```python
from build123d import *

# Parameters (mm, degrees)
F1_DEPTH = 16.256
F2_R     = 5.08
F3_W     = 14.0684605576
F3_H     = 6.096
F4_DEPTH = 10.668
F5_R     = 5.08
F6_R     = 4.8101644532
F7_DEPTH = 25.4


with BuildPart() as f1:
    # F0 (on Top) → F1 (new body)
    with BuildSketch(Plane.XY):
        Polygon((26.3900562345, 4.9985722308), (3.4010511667, 26.6430787142), (-24.288091016, 11.4677559795), (-18.4119169365, -19.5556157441), (12.9089005512, -23.5537911803), align=None)
    extrude(amount=F1_DEPTH)

    # F2
    f2_edges = [f1.edges().sort_by_distance(p)[0] for p in [
        (-18.411917, -19.555616, 8.128),
        (-2.751508, -21.554703, 0),
        (-2.751508, -21.554703, 16.256),
        (-21.350004, -4.04393, 0),
        (-10.44352, 19.055417, 0),
        (14.895554, 15.820825, 0),
        (19.649478, -9.277609, 0),
        (19.649478, -9.277609, 16.256),
        (14.895554, 15.820825, 16.256),
        (-10.44352, 19.055417, 16.256),
        (-21.350004, -4.04393, 16.256),
        (3.401051, 26.643079, 8.128),
        (-24.288091, 11.467756, 8.128),
        (12.908901, -23.553791, 8.128),
        (26.390056, 4.998572, 8.128),
    ]]
    fillet(f2_edges, radius=F2_R)

    # F3 (on face) → F4 (join)
    with BuildSketch(Plane(origin=(-21.3500039762, -4.0439298823, 0), x_dir=(0.1861022589, -0.9825303808, 0), z_dir=(-0.9825303808, -0.1861022589, 0))):
        with Locations((0.7629252505, 8.128)):
            Rectangle(F3_W, F3_H)
    extrude(amount=F4_DEPTH)

    # F5
    f5_edges = [f1.edges().sort_by_distance(p)[0] for p in [
        (-30.38057, -13.690211, 8.128),
        (-32.998742, 0.132479, 8.128),
    ]]
    fillet(f5_edges, radius=F5_R)

    # F6 (on face) → F7 (cut)
    with BuildSketch(Plane.XY.offset(11.176)):
        with Locations((-26.1089652777, -5.1103131846)):
            Circle(F6_R)
    extrude(amount=-F7_DEPTH, mode=Mode.SUBTRACT)


solid = f1.part
```
The model under review builds one solid part; all positions refer to its coordinate system, in mm. A direction names the side the tool comes from. Give positions to 0.01 mm unless a question says otherwise; leave off trailing zeros. Write each loop counter-clockwise with the first axis right and the second up, starting at its lowest first coordinate (ties: lowest second). Pieces come first, ordered by that corner, then holes. Notation, with made-up numbers: (63.5, 72.25) - (120.5, 72.25) arc R8 cw to (120.5, 80.25) - close; hole circle Ø1 at (21.25, -24.75). An arc over 180 degrees is marked (long way). Answer in a Markdown table with one row per item. Add a question column.
1. Draft analysis for pull direction Y (two halves, no side actions). For faces 1 (the cylindrical face through (13.779, 14.882, 1.528)), 2 (the flat face through (-23.067, 5.02, 8.085)), 3 (the cylindrical face through (-19.9, -3.94, 1.53)), state which applies: +Y half, -Y half, draft (parallel to the pull), parting line (faces both ways), or undercut.
2. We need section A-A on z = 9.75. Write out the cut boundary in (x, y).
3. Tool access review of faces 4 (the flat face through (-22, -8, 5.08)), 5 (the flat face through (-22, -8, 11.176)), 6 (the flat face through (-22.61, -12.22, 8.09)), 7 (the flat face through (-25.224, 1.605, 8.085)): name each direction out of +Z, -Z, +X, -X, +Y, -Y from which nothing blocks a thin tool from reaching the whole face with its end or side.
4. Insertion check: P1, Ø4, axis at y = -9.5, z = 12.5, coming from the +X side; P2, Ø1, axis at y = -9.5, z = 2, coming from the +X side; P3, Ø3.5, axis at x = -25, y = -8.5, coming from the +Z side. Each pin has a flat end and moves straight along its axis. Give the tip position at first contact, or say it passes through.
5. Wall thickness on line 1 along Y through (x, z) = (-25.5, 7.25); line 2 along Y through (x, z) = (-4.5, 2.5); line 3 along Y through (x, z) = (-6, 1.25): over which ranges is each line inside the solid? List them lowest first. Write a range as [from, to].
6. We need section B-B on z = 13.25. Write out the cut boundary in (x, y).
Ans:
| question | item | result |
|---|---|---|
| 1 | face 1 | +Y half |
| 1 | face 2 | undercut |
| 1 | face 3 | -Y half |
| 2 | outline | (-32.05, -4.86) - (-31.33, -8.7) arc R5.08 ccw to (-25.39, -12.74) - (-19.9, -11.7) - (-19.1, -15.93) arc R5.08 ccw to (-14.75, -20.02) - (9.25, -23.09) arc R5.08 ccw to (14.48, -20.22) - (24.81, 1.66) arc R5.08 ccw to (23.7, 7.53) - (6.09, 24.11) arc R5.08 ccw to (0.16, 24.87) - (-21.05, 13.24) arc R5.08 ccw to (-23.6, 7.84) - (-22.52, 2.12) - (-28.01, 1.08) arc R5.08 ccw to start; hole circle Ø9.62 at (-26.11, -5.11) |
| 3 | face 4 | -Z, -X, -Y |
| 3 | face 5 | +Z, -X, -Y |
| 3 | face 6 | +Z, -Z, -Y |
| 3 | face 7 | +Z, -Z, -X |
| 4 | P1 | stops at x = 20.39 |
| 4 | P2 | stops at x = 18.84 |
| 4 | P3 | stops at z = 11.18 |
| 5 | line 1 | y = [-12.76, -9.88], [-0.34, 1.55] |
| 5 | line 2 | y = [-20.62, 21.51] |
| 5 | line 3 | y = [-19.38, 19.5] |
| 6 | outline | (-23.17, 7.92) - (-18.66, -15.85) arc R4.64 ccw to (-14.69, -19.58) - (9.3, -22.65) arc R4.64 ccw to (14.08, -20.03) - (24.41, 1.85) arc R4.64 ccw to (23.4, 7.21) - (5.78, 23.79) arc R4.64 ccw to (0.38, 24.48) - (-20.84, 12.85) arc R4.64 ccw to start |
